from build123d import *

# Parameters (mm, degrees)
SKETCH2_W           = 600
SKETCH2_H           = 135
BOSS_EXTRUDE1_DEPTH = 8
SKETCH3_R           = 51.2
SKETCH3_W           = 150
SKETCH3_H           = 11
CUT_EXTRUDE1_DEPTH  = 8


with BuildPart() as part:
    # Sketch2 → Boss-Extrude1 (new body)
    with BuildSketch(Plane(origin=(0, 0, 0), x_dir=(1, 0, 0), z_dir=(0, 1, 0))):
        with Locations((300, 67.5)):
            Rectangle(SKETCH2_W, SKETCH2_H)
    extrude(amount=BOSS_EXTRUDE1_DEPTH)

    # Sketch3 → Cut-Extrude1 (cut)
    with BuildSketch(Plane(origin=(0, 8, 0), x_dir=(1, 0, 0), z_dir=(0, 1, 0))):
        with Locations((449.8, 67.5)):
            Circle(SKETCH3_R)
        with Locations((297.2, 67.5)):
            Circle(SKETCH3_R)
        with Locations((75, 129.5)):
            Rectangle(SKETCH3_W, SKETCH3_H)
    extrude(amount=-CUT_EXTRUDE1_DEPTH, mode=Mode.SUBTRACT)


solid = part.part
Read the model definition and answer for the solid it produces. Units are mm, in the model's axes. Give positions to 0.01 mm unless a question says otherwise; leave off trailing zeros. Write each loop counter-clockwise with the first axis right and the second up, starting at its lowest first coordinate (ties: lowest second). Pieces come first, ordered by that corner, then holes. Notation, with made-up numbers: (-1.75, 74.25) -> (21.25, 74.25) arc R21 cw to (21.25, 100.25) -> close; hole circle Ø5 at (2, -18.5). An arc over 180 degrees is marked (long way). Answer as a JSON object with one key per item and string values. Group by question number.
1) Find section D-D (z = -96). Write down the section's boundary in (x, y).
2) Consider L1, parallel to X at y = 2, z = -67.5; L2, parallel to X at y = 6, z = -43; L3, parallel to Z at x = 449.8, y = 5.5. Determine where each line is inside the solid, lowest interval first. Write a range as from..to.
3) Find section A-A (x = 297.2). Write down the section's boundary in (y, z), and give its area (3 significant figures).
4) Find section B-B (z = -67.5). Write down the section's boundary in (x, y).
5) The mould has two halves that part along X. Classify faces 1 (the flat face through (229, 0, -68)), 2 (the cylindrical face through (246.05, 4.06, -69.75)): +X half, -X half, draft (parallel to the pull), parting line (faces both ways), or undercut.
6) Find section C-C (y = 4). Write down the section's boundary in (x, z), and give its area (3 significant figures).
Values follow:
{
 "1": {"outline": "(0, 0) -> (254.67, 0) -> (254.67, 8) -> (0, 8) -> close; (339.73, 0) -> (407.27, 0) -> (407.27, 8) -> (339.73, 8) -> close; (492.33, 0) -> (600, 0) -> (600, 8) -> (492.33, 8) -> close"},
 "2": {"L1": "x = 0..246, 348.4..398.6, 501..600", "L2": "x = 0..252.24, 342.16..404.84, 494.76..600", "L3": "z = -135..-118.7, -16.3..0"},
 "3": {"outline": "(0, -135) -> (8, -135) -> (8, -118.7) -> (0, -118.7) -> close; (0, -16.3) -> (8, -16.3) -> (8, 0) -> (0, 0) -> close", "area": "261 mm2"},
 "4": {"outline": "(0, 0) -> (246, 0) -> (246, 8) -> (0, 8) -> close; (348.4, 0) -> (398.6, 0) -> (398.6, 8) -> (348.4, 8) -> close; (501, 0) -> (600, 0) -> (600, 8) -> (501, 8) -> close"},
 "5": {"face 1": "draft", "face 2": "undercut"},
 "6": {"outline": "(0, -124) -> (150, -124) -> (150, -135) -> (600, -135) -> (600, 0) -> (0, 0) -> close; hole circle Ø102.4 at (297.2, -67.5); hole circle Ø102.4 at (449.8, -67.5)", "area": "62,900 mm2"}
}
